Could you check a few things on this model? Use its own coordinates, in mm. A direction names the side the tool comes from. Round coordinates to 2 decimals unless told otherwise and drop trailing zeros. Loops run counter-clockwise (first coordinate to the right, second up) from the corner with the lowest first, then second, coordinate; pieces in that order, holes last. Notation, with made-up numbers: (77, -14.5) -> (133, -14.5) arc R25 ccw to (133, 6.5) -> close; hole circle Ø4 at (-12.5, 53). An arc over 180 degrees is marked (long way). Put each result on its own line as item: value. Start each with the question number.
1. Which directions (+Z, -Z, +X, -X, +Y, -Y) give clear straight access to the entire face, cutting with the end or side of a thin tool? Please do faces 1 (the flat face through (0, 2, 0)), 2 (the flat face through (1.588, 0, 4)).
2. I'm going to push flat-ended pins straight in: P1, Ø3, axis at x = 2.5, z = 4, coming from the +Y side; P2, Ø3, axis at x = 3.5, z = 2, coming from the -Y side; P3, Ø1.5, axis at y = 1, z = 2, coming from the +X side. Where does each tip first touch, or does it pass through?
3. Imagine slicing it at D-D, the plane z = 3. Please give me the cut outline in (x, y).
4. I need wall thicknesses on line 1 (Y direction, x = 0, z = 1.5); line 2 (Y direction, x = -1.5, z = 7.25); line 3 (X direction, y = 1.5, z = 2.5). Which ranges of each line are inside material? Lowest first, please. Write a range as [from, to].
5. Imagine slicing it at A-A, the plane z = 4. Please give me the cut outline in (x, y).
```python
from build123d import *

# Parameters (mm, degrees)
F2_SIZE  = 1.27
F3_W     = 3.175
F3_H     = 3.175
F4_DEPTH = 25.4


with BuildPart() as f1:
    # F0 (on Front) → F1 (revolve)
    with BuildSketch(Plane.XZ):
        Polygon((-6.35, 0), (0, 0), (0, 7.62), (-6.35, 7.62), (-6.35, 5.715), (-5.451974, 4.816974), (-5.900987, 4.313487), (-6.35, 4.313487), (-6.35, 3.306513), (-5.900987, 3.306513), (-5.451974, 2.803026), (-6.35, 1.905), align=None)
    revolve(axis=Axis((0, 0, 3.81), (0, 0, 1)))

    # F2
    f2_edges = [f1.edges().sort_by_distance(p)[0] for p in [
        (6.35, 0, 7.62),
        (6.35, 0, 0),
    ]]
    chamfer(f2_edges, length=F2_SIZE)

    # F3 (on face) → F4 (cut)
    with BuildSketch(Plane(origin=(0, 0, 0), x_dir=(1, 0, 0), z_dir=(0, 0, -1))):
        Rectangle(F3_W, F3_H)
    extrude(amount=-F4_DEPTH, mode=Mode.SUBTRACT)


solid = f1.part
```
Entries:
1. face 1: -Z, +X, -X, +Y, -Y
1. face 2: +Z, -Z
2. P1: y = 6.27
2. P2: y = -6.03
2. P3: x = 6.34
3. outline: circle Ø11.26 at (0, 0); hole (-1.59, -1.59) -> (1.59, -1.59) -> (1.59, 1.59) -> (-1.59, 1.59) -> close
4. line 1: [-6.35, -1.59], [1.59, 6.35]
4. line 2: [-5.24, -1.59], [1.59, 5.24]
4. line 3: [-5.56, -1.59], [1.59, 5.56]
5. outline: circle Ø12.7 at (0, 0); hole (-1.59, -1.59) -> (1.59, -1.59) -> (1.59, 1.59) -> (-1.59, 1.59) -> close
